Read the model definition and answer for the solid it produces. Units are mm, in the model's axes. Coordinates: 2 decimals unless noted, no trailing zeros. Order: outer loops, then holes, each group sorted by start corner. A loop starts at its lowest first (then second) coordinate and runs counter-clockwise, first axis right, second up. Notation, with made-up numbers: (-10.75, 45) -> (32.25, 45) arc R24 ccw to (32.25, 57) -> close; hole circle Ø4 at (-6, 23). An arc over 180 degrees is marked (long way). Return JSON: item names as keys, results as strings. Group by question number.
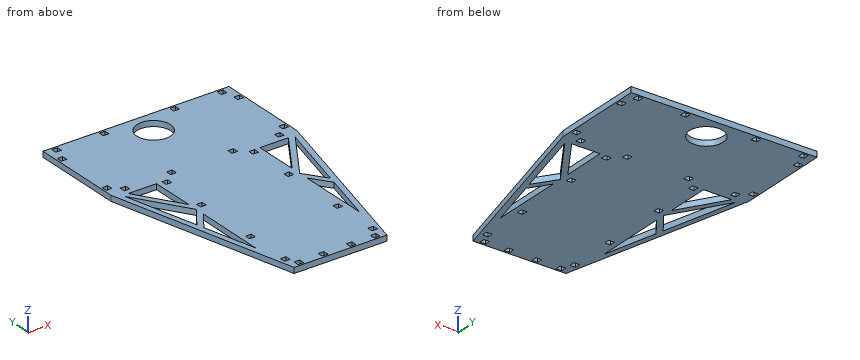
```python
from build123d import *

# Parameters (mm, degrees)
BOSS_EXTRUDE1_DEPTH = 6
SKETCH4_W           = 6
SKETCH4_H           = 6
CUT_EXTRUDE2_DEPTH  = 6
SKETCH5_R           = 18
CUT_EXTRUDE3_DEPTH  = 6


with BuildPart() as part:
    # Sketch1 → Boss-Extrude1 (new body)
    with BuildSketch(Plane.XY):
        Polygon((100, 300), (100, 200), (50, 0), (-50, 0), (-100, 200), (-100, 300), align=None)
    extrude(amount=BOSS_EXTRUDE1_DEPTH)

    # Sketch4 → Cut-Extrude2 (cut)
    with BuildSketch(Plane(origin=(0, 0, 0), x_dir=(-1, 0, 0), z_dir=(0, 0, -1))):
        with Locations((-249.21822542, 247.31110849)):
            Rectangle(SKETCH4_W, SKETCH4_H)
        with Locations((-95, 279)):
            Rectangle(SKETCH4_W, SKETCH4_H)
        with Locations((-95, 213)):
            Rectangle(SKETCH4_W, SKETCH4_H)
        with Locations((-89, 295)):
            Rectangle(SKETCH4_W, SKETCH4_H)
        with Locations((-41, 5)):
            Rectangle(SKETCH4_W, SKETCH4_H)
        with Locations((-38, 295)):
            Rectangle(SKETCH4_W, SKETCH4_H)
        with Locations((-83, 203)):
            Rectangle(SKETCH4_W, SKETCH4_H)
        with Locations((-33, 203)):
            Rectangle(SKETCH4_W, SKETCH4_H)
        with Locations((-15, 5)):
            Rectangle(SKETCH4_W, SKETCH4_H)
        with Locations((-47, 17)):
            Rectangle(SKETCH4_W, SKETCH4_H)
        with Locations((-47, 68)):
            Rectangle(SKETCH4_W, SKETCH4_H)
        with Locations((-46.748754565, 191)):
            Rectangle(SKETCH4_W, SKETCH4_H)
        with Locations((-47, 140)):
            Rectangle(SKETCH4_W, SKETCH4_H)
        with Locations((38, 295)):
            Rectangle(SKETCH4_W, SKETCH4_H)
        with Locations((89, 295)):
            Rectangle(SKETCH4_W, SKETCH4_H)
        with Locations((95, 279)):
            Rectangle(SKETCH4_W, SKETCH4_H)
        with Locations((83, 203)):
            Rectangle(SKETCH4_W, SKETCH4_H)
        with Locations((95, 213)):
            Rectangle(SKETCH4_W, SKETCH4_H)
        with Locations((46.748754565, 191)):
            Rectangle(SKETCH4_W, SKETCH4_H)
        with Locations((47, 140)):
            Rectangle(SKETCH4_W, SKETCH4_H)
        with Locations((47, 68)):
            Rectangle(SKETCH4_W, SKETCH4_H)
        with Locations((47, 17)):
            Rectangle(SKETCH4_W, SKETCH4_H)
        with Locations((41, 5)):
            Rectangle(SKETCH4_W, SKETCH4_H)
        with Locations((15, 5)):
            Rectangle(SKETCH4_W, SKETCH4_H)
        with Locations((33, 203)):
            Rectangle(SKETCH4_W, SKETCH4_H)
        Polygon((55.622098795, 194), (86.171284614, 194), (55.622098795, 146.710661579), align=None)
        Polygon((55.640072778, 135.681178614), (91.684652057, 191.47724198), (71.962334114, 112.587970208), align=None)
        Polygon((70.042546798, 104.908820946), (55.622098795, 125.311288729), (55.832173802, 48.067328963), align=None)
        Polygon((-55.832173802, 48.067328963), (-70.042546798, 104.908820946), (-55.622098795, 125.311288729), align=None)
        Polygon((-71.962334114, 112.587970208), (-55.640072778, 135.681178614), (-91.684652057, 191.47724198), align=None)
        Polygon((-86.171284614, 194), (-55.622098795, 146.710661579), (-55.622098795, 194), align=None)
    extrude(amount=-CUT_EXTRUDE2_DEPTH, mode=Mode.SUBTRACT)

    # Sketch5 → Cut-Extrude3 (cut)
    with BuildSketch(Plane(origin=(0, 0, 0), x_dir=(-1, 0, 0), z_dir=(0, 0, -1))):
        with Locations((0, 274)):
            Circle(SKETCH5_R)
    extrude(amount=-CUT_EXTRUDE3_DEPTH, mode=Mode.SUBTRACT)


solid = part.part
```
1. Find section C-C on y = 41. Determine the outline of the cut face in (x, z), and give its area (3 significant figures).
2. Given pin 1 (1.8 mm diameter, centred on y = 5, z = 2.5, fed in from +X) (3 decimals); pin 2 (1.8 mm diameter, centred on y = 15.5, z = 3.5, fed in from -X); pin 3 (3 mm diameter, centred on y = 5.5, z = 2.5, fed in from -X), each flat-ended and moving along its own axis, determine where each tip first touches the part or whether it passes through.
3. Straight lines are drawn through the part: L1, parallel to X at y = 211, z = 0.3; L2, parallel to Y at x = -35.5, z = 5.45; L3, parallel to Y at x = 0, z = 4.15. For each, find the intervals that lie inside material, in ascending order.
4. Find section A-A on x = 0. Determine the outline of the cut face in (y, z).
5. Find section B-B on z = 3.65. Give the number of separate pieces and of enclosed holes in the cut face, and give its area (3 significant figures).
Result:
{
 "1": {"outline": "(-60.25, 0) -> (60.25, 0) -> (60.25, 6) -> (-60.25, 6) -> close", "area": "723 mm^2"},
 "2": {"pin 1": "x = 51.475", "pin 2": "x = -54.1", "pin 3": "x = -51.75"},
 "3": {"L1": "-100 to -98, -92 to 92, 98 to 100", "L2": "0 to 200, 206 to 292, 298 to 300", "L3": "0 to 256, 292 to 300"},
 "4": {"outline": "(0, 0) -> (256, 0) -> (256, 6) -> (0, 6) -> close; (292, 0) -> (300, 0) -> (300, 6) -> (292, 6) -> close"},
 "5": {"separate pieces": "1", "enclosed holes": "31", "area": "43,800 mm^2"}
}
